Autodesk Inventor part; units mm, degrees
ref_plane "YZ Plane" through (0, 0, 0) normal (1, 0, 0) x (0, 1, 0)
ref_plane "XZ Plane" through (0, 0, 0) normal (0, 1, 0) x (-1, 0, 0)
ref_plane "XY Plane" through (0, 0, 0) normal (0, 0, 1) x (1, 0, 0)
ref_plane "Work Plane1" through (0, 0, 0) normal (0, 0, 1) x (1, 0, 0)
sketch "Sketch1" plane through (0, 0, 0) normal (0, 0, 1) x (1, 0, 0)
  circle A0 centre (0, 0) radius 12
  circle A1 centre (0, 0) radius 12
  circle A2 centre (0, 0) radius 15
  line L0 (0, 0) -> (0, 15)
  line L1 (0, 0) -> (-7.5, 12.9904)
  line L2 (0, 0) -> (0, -15)
  line L3 (0, 0) -> (-7.5, -12.9904)
  point P0 (-6, 10.3923)
  point P1 (-6, -10.3923)
  dimension "d0" = 24
  dimension "d1" = 30
  dimension "d2" = 30
  dimension "d3" = 30
extrude "Extrusion1" add sketch "Sketch1" against normal blind 10 contours A0 L0 A2 L2 | A0 L1 A2 L0 | L2 A2 L3 A0
sketch "Sketch2" plane through (0, 0, 0) normal (0, 0, 1) x (1, 0, 0)
  line L0 (60, -8) -> (20, -8)
  line L1 (20, -8) -> (35, -8)
  arc A0 (-7.5, -12.9904) -> (-7.5, 12.9904) centre (0, 0) ccw
  line L2 (20, -8) -> (12.6886, -8)
  line L3 (35, -8) -> (35, 8)
  line L4 (35, 8) -> (20, 8)
  line L5 (20, 8) -> (12.6886, 8)
  line L6 (35, -8) -> (35, -4)
  line L7 (35, -4) -> (14.4568, -4)
  line L8 (35, 8) -> (35, 4)
  line L9 (35, 4) -> (14.4568, 4)
  dimension "d6" = 15
  dimension "d7" = 16
  dimension "d8" = 15
  dimension "d9" = 4
  dimension "d10" = 4
extrude "Extrusion2" add sketch "Sketch2" against normal up to surface (10 mm away) contours L0 L2 A0 L7 L3 | L9 A0 L5 L4 L3
fillet "Fillet1" radius 15 2 edges at (12.6886, 8, -5) (12.6886, -8, -5)
thicken "Thicken1" operation add thickness 2 both sides no extend neighbours yes toward (0.9780418, 0.2084088, 0) faces at (14.6706, 3.1261, -6.6667)
fillet "Fillet2" radius 2 2 edges at (16.5227, 4, -5) (16.5227, -4, -5)
thicken "Thicken2" operation add thickness 2 both sides no extend neighbours yes toward (1, 0, 0) faces at (35, -6.6667, -3.3333)
thicken "Thicken3" operation add thickness 2 both sides no extend neighbours yes toward (1, 0, 0) faces at (35, 6.6667, -6.6667)
sketch "Sketch4" plane through (19.2614, -8, -10) normal (0, -1, 0) x (1, 0, 0)
  line L0 (0, 0) -> (0, 10)
  line L1 (17.7386, 0) -> (0, 0)
  line L2 (17.7386, 10) -> (17.7386, 0)
  line L3 (0, 10) -> (17.7386, 10)
  line L4 (0, 10) -> (0, 0)
  line L5 (0, 5) -> (5, 5)
  line L6 (5, 5) -> (13, 5)
  circle A0 centre (5, 5) radius 1.5
  circle A1 centre (13, 5) radius 1.5
  point P0 (-19.2614, 10)
  dimension "d30" = 5
  dimension "d31" = 8
  dimension "d32" = 3
  dimension "d33" = 3
extrude "Extrusion4" cut sketch "Sketch4" against normal up to surface (16 mm away) contours A0 L6 L5 | L5 L6 A0 | A1
chamfer "Chamfer1" distance 2 angle 45 4 edges at (37, -6, -10) (37, 6, 0) (37, -6, 0) (37, 6, -10)
chamfer "Chamfer2" distance 2 angle 45 4 edges at (-6.75, -11.6913, -10) (-6.75, -11.6913, 0) (-6.75, 11.6913, 0) (-6.75, 11.6913, -10)
fillet "Fillet4" radius 3 4 edges at (-4.9425, -12.5607, -10) (-4.9425, 12.5607, -10) (-4.9425, -12.5607, 0) (-4.9425, 12.5607, 0)
sketch "Sketch5" plane through (18.8944, 4, -10) normal (0, -1, 0) x (1, 0, 0)
  line L0 (16.1056, 10) -> (18.1056, 8)
  line L1 (0.3669, 10) -> (16.1056, 10)
  line L2 (0.3669, 0) -> (0.3669, 10)
  line L3 (16.1056, 0) -> (0.3669, 0)
  line L4 (18.1056, 2) -> (16.1056, 0)
  line L5 (18.1056, 8) -> (18.1056, 2)
  circle A0 centre (5.3669, 5) radius 1.5
  circle A1 centre (13.3669, 5) radius 1.5
  line L6 (0.3669, 10) -> (16.1056, 10)
  line L7 (16.1056, 10) -> (10.1056, 10)
  line L8 (10.1056, 10) -> (10.1056, 0)
  point P0 (-18.8944, 10)
  point P1 (10.1056, 10)
  point P2 (10.1056, 0)
  dimension "d43" = 6
extrude "Extrusion5" add sketch "Sketch5" along normal up to surface (8 mm away) contours L0 L5 L4 L3 L8 L1
chamfer "Chamfer3" distance 2 angle 45 2 edges at (29, 0, -10) (29, 0, 0)
fillet "Fillet5" radius 2 6 edges at (30, -4, -1) (29, -4, -5) (30, -4, -9) (30, 4, -9) (29, 4, -5) (30, 4, -1)
properties part number "motor_holder_1"
Design review of the part built by this model. Coordinates are the model's own, in mm. A direction names the side the tool comes from. Coordinates: 2 decimals unless noted, no trailing zeros. Loops run counter-clockwise (first coordinate to the right, second up) from the corner with the lowest first, then second, coordinate; pieces in that order, holes last. Notation, with made-up numbers: M 28,22 L 59,22 A27 ccw 59,48 Z; hole C 38.25,39.5 d7. An arc over 180 degrees is marked long. One line per question, with ' | ' between items.
(1) Machinability: for faces 1 (the face through (-6.23, 11.93, -8.57)), 2 (the face through (-6.739, 11.673, -4.958)), 3 (the face through (29.3, 3.43, -9.15)), 4 (the face through (17.423, 3.355, -4.93)), which of the approach directions +Z, -Z, +X, -X, +Y, -Y give a long, thin tool a straight path to every point of the face, cutting with its end or side? Answer none if there is none.
Filled in:
face 1: -Z, -X | face 2: +Z, -Z, -X | face 3: -Z | face 4: +Z, -Z
(2) We need section A-A (x = 0). Give the boundary of the cut face in (y, z).
Filled in:
outline: M -15,-10 L -12,-10 L -12,0 L -15,0 Z; M 12,-10 L 15,-10 L 15,0 L 12,0 Z
(3) We need section C-C (z = -7.5). Give the boundary of the cut face in (x, y), and give its area (3 significant figures).
Filled in:
outline: M -7.5,-12.99 A15 ccw 9.63,-11.5 A15 cw 19.26,-8 L 37,-8 L 37,8 L 19.26,8 A15 cw 9.63,11.5 A15 ccw -7.5,12.99 L -6,10.39 A12 cw long -6,-10.39 Z; hole M 16.91,-1.79 A2 ccw 18.89,-4 L 27,-4 A2 ccw 29,-2 L 29,2 A2 ccw 27,4 L 18.89,4 A2 ccw 16.91,1.79 A17 cw Z | area: 450 mm^2
(4) We need section D-D (y = -6). Give the boundary of the cut face in (x, z), and give its area (3 significant figures).
Filled in:
outline: M 10.39,-10 L 35,-10 L 37,-8 L 37,-2 L 35,0 L 10.39,0 Z; hole C 24.26,-5 d3; hole C 32.26,-5 d3 | area: 248 mm^2
(5) Wall thickness on probe 1 along Y at (x, z) = (26.5, -8.5); probe 2 along Y at (x, z) = (0, -5.5); probe 3 along Y at (x, z) = (30, -1.5): over which ranges is each line inside the solid? List them lowest first.
Filled in:
probe 1: y = -8 to -4, 4 to 8 | probe 2: y = -15 to -12, 12 to 15 | probe 3: y = -8 to 8
(6) Draft analysis for pull direction Z (two halves, no side actions). For faces 5 (the face through (25.692, 5.972, -4.549)), 6 (the face through (-4.839, 12.54, -0.235)), 7 (the face through (17.39, -3.32, -4.93)), state which applies: released by +Z, released by -Z, zero draft, split by the parting line, or undercut.
Filled in:
face 5: undercut | face 6: released by +Z | face 7: zero draft
(7) For pin 1 Ø3.5 at (x, z) = (32.26, -5) entering from -Y; pin 2 Ø4 at (y, z) = (-2, -9) entering from -X; pin 3 Ø3.5 at (x, z) = (24.26, -5) entering from +Y, all flat-tipped, find the tip position at first contact; note any pin that passes through.
Filled in:
pin 1: stops at y = -8 | pin 2: stops at x = 11.31 | pin 3: stops at y = 8
(8) We need section B-B (y = 0). Give the boundary of the cut face in (x, z), and give its area (3 significant figures).
Filled in:
outline: M 12,-10 L 17,-10 L 17,0 L 12,0 Z; M 29,-8 L 31,-10 L 35,-10 L 37,-8 L 37,-2 L 35,0 L 31,0 L 29,-2 Z; hole C 32.26,-5 d3 | area: 115 mm^2
